```python
from build123d import *

# Parameters (mm, degrees)
BOSS_EXTRUDE1_DEPTH = 15
SKETCH1_7_R         = 7.5
BOSS_EXTRUDE5_DEPTH = 15


with BuildPart() as part:
    # Sketch1 → Boss-Extrude1 (new body)
    with BuildSketch(Plane.XY):
        Polygon((60, -32.5), (60, -27.5), (-60, 4.653903092), (-60, -32.5), align=None)
    extrude(amount=BOSS_EXTRUDE1_DEPTH)

    # Sketch1_7 → Boss-Extrude5 (add)
    with BuildSketch(Plane.XY):
        Polygon((5.548089225, 32.5), (-60, 32.5), (-60, -32.5), (60, -32.5), (60, 10.5), align=None)
        with Locations((-32, 20.5)):
            Circle(SKETCH1_7_R, mode=Mode.SUBTRACT)
        with Locations((35, 2.5)):
            Circle(SKETCH1_7_R, mode=Mode.SUBTRACT)
    extrude(amount=-BOSS_EXTRUDE5_DEPTH)


solid = part.part
```
Design review of the part built by this model. Coordinates are the model's own, in mm. A direction names the side the tool comes from. Round coordinates to 2 decimals unless told otherwise and drop trailing zeros. Write each loop counter-clockwise with the first axis right and the second up, starting at its lowest first coordinate (ties: lowest second). Pieces come first, ordered by that corner, then holes. Notation, with made-up numbers: (-4, 54.25) -> (47, 54.25) arc R23 ccw to (47, 84.25) -> close; hole circle Ø7 at (-30, 18.5). An arc over 180 degrees is marked (long way). Answer in a Markdown table with one row per item.
Q1. Draft analysis for pull direction X (two halves, no side actions). For faces 3 (the face through (-1, 10, 0)), 4 (the face through (27.507, 2.83, -7.395)), 5 (the face through (33.155, 21.346, -7.395)), state which applies: +X half, -X half, draft (parallel to the pull), parting line (faces both ways), or undercut.
The answers:
| item | result |
|---|---|
| face 3 | draft |
| face 4 | undercut |
| face 5 | +X half |
Q2. For faces 1 (the face through (60, -11, -6)), 2 (the face through (0.84, -11.65, 7.4)), list the 3-axis set-ups (+Z, -Z, +X, -X, +Y, -Y) from which the entire face can be reached by the end or side of a thin tool; tool diameter is ignored.
The answers:
| item | result |
|---|---|
| face 1 | +Z, -Z, +X, +Y, -Y |
| face 2 | +Z, +X, +Y |
Q3. Take a section at B-B, the plane y = 2.5. State the section outline as (x, z) points, then the cut area to 3 significant figures.
The answers:
| item | result |
|---|---|
| outline | (-60, -15) -> (27.5, -15) -> (27.5, 0) -> (-51.96, 0) -> (-51.96, 15) -> (-60, 15) -> close; (42.5, -15) -> (60, -15) -> (60, 0) -> (42.5, 0) -> close |
| area | 1,700 mm² |
Q4. Take a section at C-C, the plane x = -32. State the section outline as (y, z) points.
The answers:
| item | result |
|---|---|
| outline | (-32.5, -15) -> (13, -15) -> (13, 0) -> (-2.85, 0) -> (-2.85, 15) -> (-32.5, 15) -> close; (28, -15) -> (32.5, -15) -> (32.5, 0) -> (28, 0) -> close |
Q5. To check wall thickness, follow L1, parallel to Y at x = -32, z = -4.25; L2, parallel to Z at x = -41, y = 27.5; L3, parallel to Y at x = -34, z = -9. State the ranges of each line that lie inside material, in increasing order. Write a range as [from, to].
The answers:
| item | result |
|---|---|
| L1 | [-32.5, 13], [28, 32.5] |
| L2 | [-15, 0] |
| L3 | [-32.5, 13.27], [27.73, 32.5] |
Q6. Take a section at D-D, the plane x = -50.5. State the section outline as (y, z) points, then the cut area to 3 significant figures.
The answers:
| item | result |
|---|---|
| outline | (-32.5, -15) -> (32.5, -15) -> (32.5, 0) -> (2.11, 0) -> (2.11, 15) -> (-32.5, 15) -> close |
| area | 1,490 mm² |
Q7. Take a section at A-A, the plane z = -3.75. State the section outline as (x, y) points.
The answers:
| item | result |
|---|---|
| outline | (-60, -32.5) -> (60, -32.5) -> (60, 10.5) -> (5.55, 32.5) -> (-60, 32.5) -> close; hole circle Ø15 at (-32, 20.5); hole circle Ø15 at (35, 2.5) |
Q8. Clearance check with flat-ended pins moving along their axes: pin 1 Ø24 at (x, y) = (35, 2.5) entering from -Z; pin 2 Ø18 at (x, y) = (18, 11) entering from +Z; pin 3 Ø6 at (y, z) = (8.5, 11) entering from +X. State where each tip first meets the part, or that it passes through.
The answers:
| item | result |
|---|---|
| pin 1 | z = -15 |
| pin 2 | z = 0 |
| pin 3 | through |
